The listing builds one solid part. Answer for the finished solid, in the listing's coordinates (mm). Face numbers are marked on the shaded views. Give positions to 0.01 mm unless a question says otherwise; leave off trailing zeros. Write each loop counter-clockwise with the first axis right and the second up, starting at its lowest first coordinate (ties: lowest second). Pieces come first, ordered by that corner, then holes. Notation, with made-up numbers: (51.25, 80.25) - (82.25, 80.25) arc R18 ccw to (82.25, 93.25) - close; hole circle Ø8 at (44.25, -33). An arc over 180 degrees is marked (long way). Return JSON: item names as keys, results as strings.
from build123d import *

# Parameters (mm, degrees)
F0_W     = 300
F0_H     = 450
F0_W_2   = 219
F0_H_2   = 48
F0_H_3   = 54
F0_W_3   = 63
F0_H_4   = 438
F0_W_4   = 69
F0_H_5   = 324
F1_DEPTH = 48


with BuildPart() as f1:
    # F0 (on Top) → F1 (new body)
    with BuildSketch(Plane.XY):
        Rectangle(F0_W, F0_H)
        with Locations((34.5, -195)):
            Rectangle(F0_W_2, F0_H_2, mode=Mode.SUBTRACT)
        with Locations((34.5, -138)):
            Rectangle(F0_W_2, F0_H_3, mode=Mode.SUBTRACT)
        with Locations((-112.5, 0)):
            Rectangle(F0_W_3, F0_H_4, mode=Mode.SUBTRACT)
        with Locations((-40.5, 57)):
            Rectangle(F0_W_4, F0_H_5, mode=Mode.SUBTRACT)
        with Locations((34.5, 57)):
            Rectangle(F0_W_4, F0_H_5, mode=Mode.SUBTRACT)
        with Locations((109.5, 57)):
            Rectangle(F0_W_4, F0_H_5, mode=Mode.SUBTRACT)
    extrude(amount=F1_DEPTH)


solid = f1.part
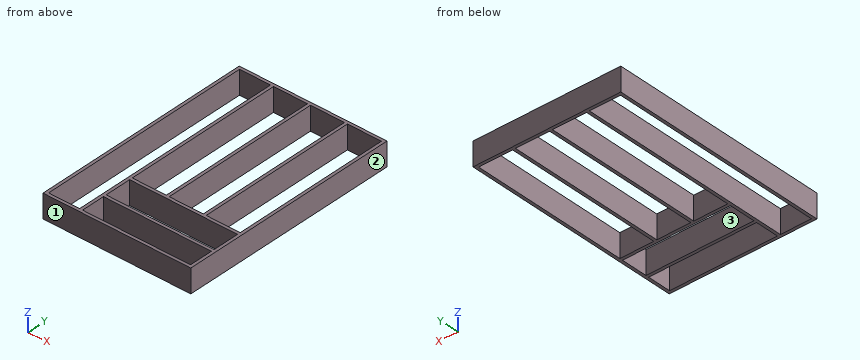
Item 1: A cutting plane is placed at B-B on x = -103. Determine the outline of the cut face in (y, z), then the cut area to 3 significant figures.
Answer below:
{"outline": "(-225, 0) - (-219, 0) - (-219, 48) - (-225, 48) - close; (219, 0) - (225, 0) - (225, 48) - (219, 48) - close", "area": "576 mm²"}
Item 2: Consider L1, parallel to X at y = 93.5, z = 33.5; L2, parallel to Y at x = -25, z = 3.5; L3, parallel to X at y = -182.5, z = 26.5. Determine where each line is inside the solid, lowest interval first.
Answer below:
{"L1": "x = -150 to -144, -81 to -75, -6 to 0, 69 to 75, 144 to 150", "L2": "y = -225 to -219, -171 to -165, -111 to -105, 219 to 225", "L3": "x = -150 to -144, -81 to -75, 144 to 150"}
Item 3: A cutting plane is placed at D-D on z = 26. Determine the outline of the cut face in (x, y).
Answer below:
{"outline": "(-150, -225) - (150, -225) - (150, 225) - (-150, 225) - close; hole (-144, -219) - (-81, -219) - (-81, 219) - (-144, 219) - close; hole (-75, -219) - (144, -219) - (144, -171) - (-75, -171) - close; hole (-75, -165) - (144, -165) - (144, -111) - (-75, -111) - close; hole (-75, -105) - (-6, -105) - (-6, 219) - (-75, 219) - close; hole (0, -105) - (69, -105) - (69, 219) - (0, 219) - close; hole (75, -105) - (144, -105) - (144, 219) - (75, 219) - close"}
Item 4: A cutting plane is placed at C-C on x = 93. Determine the outline of the cut face in (y, z).
Answer below:
{"outline": "(-225, 0) - (-219, 0) - (-219, 48) - (-225, 48) - close; (-171, 0) - (-165, 0) - (-165, 48) - (-171, 48) - close; (-111, 0) - (-105, 0) - (-105, 48) - (-111, 48) - close; (219, 0) - (225, 0) - (225, 48) - (219, 48) - close"}
Item 5: The mould has two halves that part along Y. Classify the marked faces 1, 2 and 3: +Y half, -Y half, draft (parallel to the pull), parting line (faces both ways), or undercut.
Answer below:
{"face 1": "-Y half", "face 2": "draft", "face 3": "undercut"}
Item 6: A cutting plane is placed at A-A on y = -13.5. Determine the outline of the cut face in (x, z).
Answer below:
{"outline": "(-150, 0) - (-144, 0) - (-144, 48) - (-150, 48) - close; (-81, 0) - (-75, 0) - (-75, 48) - (-81, 48) - close; (-6, 0) - (0, 0) - (0, 48) - (-6, 48) - close; (69, 0) - (75, 0) - (75, 48) - (69, 48) - close; (144, 0) - (150, 0) - (150, 48) - (144, 48) - close"}
